```python
from build123d import *

# Parameters (mm, degrees)
SKETCH_1_W          = 6
SKETCH_1_H          = 6
EXTRUDE_1_DEPTH     = 0.5
SKETCH_2_W          = 3.9
SKETCH_2_H          = 3.9
CUT_EXTRUDE_1_DEPTH = 5.272001873
SKETCH_3_W          = 4.2
SKETCH_3_H          = 4.2
CUT_EXTRUDE_2_DEPTH = 0.3
SKETCH_4_W          = 0.8
SKETCH_4_H          = 0.8
CUT_EXTRUDE_3_DEPTH = 5.272001873
FILLET_2_R          = 0.2


with BuildPart() as part:
    # 草图1 → 凸台-拉伸1 (new body)
    with BuildSketch(Plane(origin=(0, 0, 0), x_dir=(1, 0, 0), z_dir=(0, 1, 0))):
        Rectangle(SKETCH_1_W, SKETCH_1_H)
    extrude(amount=EXTRUDE_1_DEPTH)

    # 草图2 → 切除-拉伸1 (cut, through all)
    with BuildSketch(Plane(origin=(0, 0.5, 0), x_dir=(1, 0, 0), z_dir=(0, 1, 0))):
        Rectangle(SKETCH_2_W, SKETCH_2_H)
    extrude(amount=-CUT_EXTRUDE_1_DEPTH, mode=Mode.SUBTRACT)

    # 草图3 → 切除-拉伸2 (cut)
    with BuildSketch(Plane(origin=(0, 0.5, 0), x_dir=(1, 0, 0), z_dir=(0, 1, 0))):
        Rectangle(SKETCH_3_W, SKETCH_3_H)
    extrude(amount=-CUT_EXTRUDE_2_DEPTH, mode=Mode.SUBTRACT)

    # 草图4 → 切除-拉伸3 (cut, through all)
    with BuildSketch(Plane(origin=(0, 0.5, 0), x_dir=(1, 0, 0), z_dir=(0, 1, 0))):
        with Locations((-2.6, 2.6)):
            Rectangle(SKETCH_4_W, SKETCH_4_H)
        with Locations((2.6, 2.6)):
            Rectangle(SKETCH_4_W, SKETCH_4_H)
        with Locations((-2.6, -2.6)):
            Rectangle(SKETCH_4_W, SKETCH_4_H)
        with Locations((2.6, -2.6)):
            Rectangle(SKETCH_4_W, SKETCH_4_H)
    extrude(amount=-CUT_EXTRUDE_3_DEPTH, mode=Mode.SUBTRACT)

    # 圆角2
    fillet_2_edges = [part.edges().sort_by_distance(p)[0] for p in [
        (-2.2, 0.25, -2.2),
        (2.2, 0.25, -2.2),
        (-2.2, 0.25, 2.2),
        (2.2, 0.25, 2.2),
    ]]
    fillet(fillet_2_edges, radius=FILLET_2_R)


solid = part.part
```
Model file for the job. Use its own axes, mm. Round coordinates to 2 decimals unless told otherwise and drop trailing zeros. Write each loop counter-clockwise with the first axis right and the second up, starting at its lowest first coordinate (ties: lowest second). Pieces come first, ordered by that corner, then holes. Notation, with made-up numbers: (-5, 29.5) - (51, 29.5) arc R8 ccw to (51, 40.5) - close; hole circle Ø7 at (-31.5, 13). An arc over 180 degrees is marked (long way). One line per item, written item: value.
(1) Cut at B-B, the plane x = -0.4. Give the cut face in (y, z).
Values follow:
outline: (0, -3) - (0.5, -3) - (0.5, -2.1) - (0.2, -2.1) - (0.2, -1.95) - (0, -1.95) - close; (0, 1.95) - (0.2, 1.95) - (0.2, 2.1) - (0.5, 2.1) - (0.5, 3) - (0, 3) - close
(2) Wall check: probe 1 along X at (y, z) = (0.45, -0.65); probe 2 along Z at (x, y) = (-1.75, 0.1). Give the ranges that are in metal, low to high.
Values follow:
probe 1: x = -3 to -2.1, 2.1 to 3
probe 2: z = -3 to -1.95, 1.95 to 3
(3) Drop a flat-ended pin along its axis: P1, Ø2, axis at x = -0.5, z = -1, coming from the +Y side. Give the stop position or say it passes through.
Values follow:
P1: stops at y = 0.2
(4) Cut at D-D, the plane z = -2.5. Give the cut face in (x, y).
Values follow:
outline: (-2.2, 0) - (2.2, 0) - (2.2, 0.5) - (-2.2, 0.5) - close
(5) Cut at A-A, the plane z = -0.15. Give the cut face in (x, y), plus the area to 3 significant figures.
Values follow:
outline: (-3, 0) - (-1.95, 0) - (-1.95, 0.2) - (-2.1, 0.2) - (-2.1, 0.5) - (-3, 0.5) - close; (1.95, 0) - (3, 0) - (3, 0.5) - (2.1, 0.5) - (2.1, 0.2) - (1.95, 0.2) - close
area: 0.960 mm²
(6) Cut at C-C, the plane y = 0.35. Give the cut face in (x, z).
Values follow:
outline: (-3, -2.2) - (-2.4, -2.2) arc R0.2 cw to (-2.2, -2.4) - (-2.2, -3) - (2.2, -3) - (2.2, -2.4) arc R0.2 cw to (2.4, -2.2) - (3, -2.2) - (3, 2.2) - (2.4, 2.2) arc R0.2 cw to (2.2, 2.4) - (2.2, 3) - (-2.2, 3) - (-2.2, 2.4) arc R0.2 cw to (-2.4, 2.2) - (-3, 2.2) - close; hole (-2.1, -2.1) - (2.1, -2.1) - (2.1, 2.1) - (-2.1, 2.1) - close
